```python
from build123d import *

# Parameters (mm, degrees)
F0_W     = 210
F0_H     = 25
F1_DEPTH = 25
F2_R     = 4
F3_DEPTH = 25.001
F4_R     = 10
F5_DEPTH = 110


with BuildPart() as f1:
    # F0 (on Top) → F1 (new body)
    with BuildSketch(Plane.XY):
        Rectangle(F0_W, F0_H)
    extrude(amount=F1_DEPTH)

    # F2 (on face) → F3 (cut, through all)
    with BuildSketch(Plane.XZ.offset(12.5)):
        with Locations((-95, 12.5)):
            Circle(F2_R)
        with Locations((15, 12.5)):
            Circle(F2_R)
    extrude(amount=-F3_DEPTH, mode=Mode.SUBTRACT)

    # F4 (on face) → F5 (cut)
    with BuildSketch(Plane.YZ.offset(105)):
        with Locations((0, 12.5)):
            Circle(F4_R)
    extrude(amount=-F5_DEPTH, mode=Mode.SUBTRACT)


solid = f1.part
```
Verification items for the finished model (mm, model axes). A direction names the side the tool comes from. Round coordinates to 2 decimals unless told otherwise and drop trailing zeros. Order: outer loops, then holes, each group sorted by start corner. A loop starts at its lowest first (then second) coordinate and runs counter-clockwise, first axis right, second up.
1) Cross-section at D-D, the plane x = 40.5. Record the cut outline in (y, z), plus the area to 3 significant figures.
Geometry says:
outline: (-12.5, 0) - (12.5, 0) - (12.5, 25) - (-12.5, 25) - close; hole circle Ø20 at (0, 12.5)
area: 311 mm2
2) Cross-section at B-B, the plane y = 0. Record the cut outline in (x, z), plus the area to 3 significant figures.
Geometry says:
outline: (-105, 0) - (105, 0) - (105, 2.5) - (-5, 2.5) - (-5, 22.5) - (105, 22.5) - (105, 25) - (-105, 25) - close; hole circle Ø8 at (-95, 12.5)
area: 3,000 mm2
3) Cross-section at A-A, the plane x = 15. Record the cut outline in (y, z).
Geometry says:
outline: (-12.5, 0) - (12.5, 0) - (12.5, 8.5) - (9.17, 8.5) arc R10 cw to (-9.17, 8.5) - (-12.5, 8.5) - close; (-12.5, 16.5) - (-9.17, 16.5) arc R10 cw to (9.17, 16.5) - (12.5, 16.5) - (12.5, 25) - (-12.5, 25) - close
4) Tool access check on faces 4 (the cylindrical face through (12.05, 11.18, 15.2)), 5 (the flat face through (-5, 0, 13)). Record the directions out of +Z, -Z, +X, -X, +Y, -Y that give a thin tool (end or side, any length) a straight path to the whole face; none if there is none.
Geometry says:
face 4: +Y, -Y
face 5: +X
5) Cross-section at C-C, the plane z = 12.5. Record the cut outline in (x, y), plus the area to 3 significant figures.
Geometry says:
outline: (-105, -12.5) - (-99, -12.5) - (-99, 12.5) - (-105, 12.5) - close; (-91, -12.5) - (11, -12.5) - (11, -10) - (-5, -10) - (-5, 10) - (11, 10) - (11, 12.5) - (-91, 12.5) - close; (19, -12.5) - (105, -12.5) - (105, -10) - (19, -10) - close; (19, 10) - (105, 10) - (105, 12.5) - (19, 12.5) - close
area: 2,810 mm2
6) Depth check by flat-ended pin: pin 1 (13 mm diameter, centred on x = 15, z = 12.5, fed in from +Y); pin 2 (5 mm diameter, centred on y = -4, z = 7.5, fed in from +X). Enter the tip coordinate at first touch or a pass-through.
Geometry says:
pin 1: stops at y = 12.5
pin 2: stops at x = -5
7) Material ranges on line 1 (Y direction, x = 47, z = 12.5); line 2 (Z direction, x = 15, y = 11.1); line 3 (Y direction, x = 11, z = 16.5), recorded low to high.
Geometry says:
line 1: y = -12.5 to -10, 10 to 12.5
line 2: z = 0 to 8.5, 16.5 to 25
line 3: y = -12.5 to -9.17, 9.17 to 12.5
8) Draft check along Y on faces 1 (the flat face through (-1, 12.5, 12)), 2 (the cylindrical face through (50.77, -9.99, 12.94)), 3 (the flat face through (105, -9, 7)). Enter one of: +Y half, -Y half, draft (parallel to the pull), parting line (faces both ways), or undercut.
Geometry says:
face 1: +Y half
face 2: undercut
face 3: draft
